Autodesk Inventor part; units mm, degrees
ref_plane "YZ Plane" through (0, 0, 0) normal (1, 0, 0) x (0, 1, 0)
ref_plane "XZ Plane" through (0, 0, 0) normal (0, 1, 0) x (-1, 0, 0)
ref_plane "XY Plane" through (0, 0, 0) normal (0, 0, 1) x (1, 0, 0)
sketch "Sketch1" plane through (0, 0, 0) normal (0, 1, 0) x (-1, 0, 0)
  line L0 (-43.2, 43.2) -> (43.2, 43.2)
  line L1 (43.2, 43.2) -> (43.2, -43.2)
  line L2 (43.2, -43.2) -> (-43.2, -43.2)
  line L3 (-43.2, -43.2) -> (-43.2, 43.2)
  line L4 (-43.2, 43.2) -> (43.2, -43.2) construction
  line L5 (43.2, 43.2) -> (-43.2, -43.2) construction
  point P0 (0, 0)
  dimension "d0" = 86.4
  dimension "d1" = 86.4
extrude "Extrusion1" add sketch "Sketch1" along normal blind 3
sketch "Sketch2" plane through (0, 3, 0) normal (0, 1, 0) x (1, 0, 0)
  line L0 (-43.2, -43.2) -> (43.2, -43.2)
  line L1 (-43.2, -43.2) -> (-11.2, -43.2)
  line L2 (-11.2, -23) -> (-43.2, -23)
  line L3 (-43.2, -23) -> (-43.2, 23)
  line L4 (-43.2, 23) -> (-11.2, 23)
  line L5 (-11.2, 23) -> (-11.2, -23)
  line L6 (-11.2, -23) -> (-43.2, 23) construction
  line L7 (-43.2, -23) -> (-11.2, 23) construction
  point P0 (0, 0)
  point P1 (-27.2, 0)
  dimension "d5" = 46
extrude "Extrusion2" add sketch "Sketch2" along normal blind 46
scale "Scale1" factors (0.5, 0.5, 0.5) then translate (0, 0, 0) bodies 1
properties part number "DCDriver"
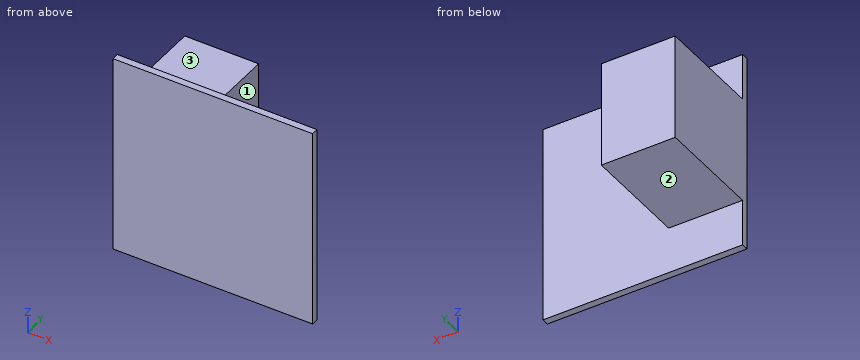
Design review of the part built by this model. Coordinates are the model's own, in mm. Face numbers are marked on the shaded views. A direction names the side the tool comes from. Coordinates: 2 decimals unless noted, no trailing zeros. Loops run counter-clockwise (first coordinate to the right, second up) from the corner with the lowest first, then second, coordinate; pieces in that order, holes last. Notation, with made-up numbers: (69.5, 41.5) - (97.5, 41.5) arc R21 cw to (97.5, 46.5) - close; hole circle Ø8 at (58.25, -2). An arc over 180 degrees is marked (long way). Use CSV: the item, a comma, the result in double quotes. Start each with the question number.
1. Clearance check with flat-ended pins moving along their axes: pin 1 (1 mm diameter, centred on x = 12, z = -7.5, fed in from +Y); pin 2 (12 mm diameter, centred on y = 11, z = -11.5, fed in from +X); pin 3 (13 mm diameter, centred on x = -13.5, y = 11.5, fed in from +Z). State where each tip first meets the part, or that it passes through.
2. To check wall thickness, follow probe 1 along X at (y, z) = (17, -9); probe 2 along Y at (x, z) = (17, -12.5); probe 3 along Z at (x, y) = (-10.5, 2.75). State the ranges of each line that lie inside material, in increasing order.
3. Add section C-C on y = 5. Give the boundary of the cut face in (x, z), plus the area to 3 significant figures.
4. Add section B-B on z = 10.5. Give the boundary of the cut face in (x, y).
5. Add section D-D on x = 2.5. Give the boundary of the cut face in (y, z).
6. Add section A-A on x = -12.5. Give the boundary of the cut face in (y, z), plus the area to 3 significant figures.
7. For the marked faces 1, 2 and 3, list the 3-axis set-ups (+Z, -Z, +X, -X, +Y, -Y) from which the entire face can be reached by the end or side of a thin tool; tool diameter is ignored.
Resolved:
1,pin 1,"y = 1.5"
1,pin 2,"x = -5.6"
1,pin 3,"z = 11.5"
2,probe 1,"-21.6 to -5.6"
2,probe 2,"0 to 1.5"
2,probe 3,"-11.5 to 11.5"
3,outline,"(-21.6, -11.5) - (-5.6, -11.5) - (-5.6, 11.5) - (-21.6, 11.5) - close"
3,area,"368 mm2"
4,outline,"(-21.6, 0) - (21.6, 0) - (21.6, 1.5) - (-5.6, 1.5) - (-5.6, 24.5) - (-21.6, 24.5) - close"
5,outline,"(0, -21.6) - (1.5, -21.6) - (1.5, 21.6) - (0, 21.6) - close"
6,outline,"(0, -21.6) - (1.5, -21.6) - (1.5, -11.5) - (24.5, -11.5) - (24.5, 11.5) - (1.5, 11.5) - (1.5, 21.6) - (0, 21.6) - close"
6,area,"594 mm2"
7,face 1,"+Z, -Z, +X, +Y"
7,face 2,"-Z, +X, -X, +Y"
7,face 3,"+Z, +X, -X, +Y"
